Can you work these out from the model? Positions are in its coordinate system, mm. Coordinates: 2 decimals unless noted, no trailing zeros. Write each loop counter-clockwise with the first axis right and the second up, starting at its lowest first coordinate (ties: lowest second). Pieces come first, ordered by that corner, then holes. Notation, with made-up numbers: (-20, 81.5) -> (25, 81.5) arc R26 ccw to (25, 98.5) -> close; hole circle Ø6 at (-26, -16.75). An arc over 180 degrees is marked (long way). Use one line per item in the form item = value.
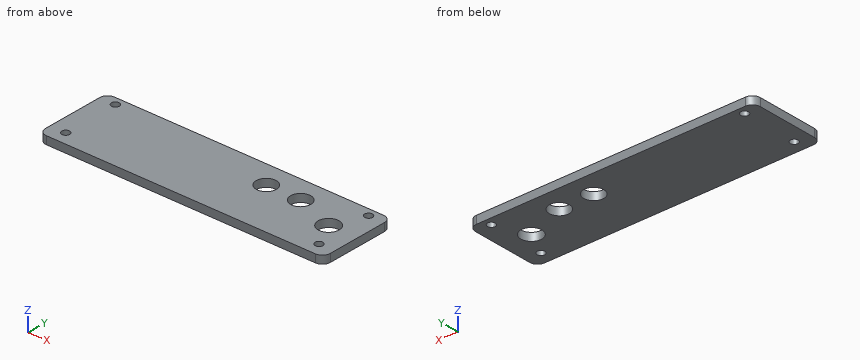
```python
from build123d import *

# Parameters (mm, degrees)
F0_R     = 1.5
F0_R_2   = 3.825
F1_DEPTH = 3


with BuildPart() as f1:
    # F0 (on Top) → F1 (new body)
    with BuildSketch(Plane.XY):
        with BuildLine():
            Line((54.25, -11.75), (54.25, 0))
            Line((54.25, 0), (47.317251, 0))
            ThreePointArc((47.317251, 0), (43.317251, -4), (39.317251, 0))
            Line((39.317251, 0), (-54.25, 0))
            Line((-54.25, 0), (-54.25, -11.75))
            ThreePointArc((-54.25, -11.75), (-53.37132, -13.87132), (-51.25, -14.75))
            Line((-51.25, -14.75), (51.25, -14.75))
            ThreePointArc((51.25, -14.75), (53.37132, -13.87132), (54.25, -11.75))
        make_face()
        with Locations((-48.25, -9.8)):
            Circle(F0_R, mode=Mode.SUBTRACT)
        with Locations((48.25, -9.8)):
            Circle(F0_R, mode=Mode.SUBTRACT)
        with BuildLine():
            ThreePointArc((54.25, 11.75), (53.37132, 13.87132), (51.25, 14.75))
            Line((51.25, 14.75), (-51.25, 14.75))
            ThreePointArc((-51.25, 14.75), (-53.37132, 13.87132), (-54.25, 11.75))
            Line((-54.25, 11.75), (-54.25, 0))
            Line((-54.25, 0), (39.317251, 0))
            ThreePointArc((39.317251, 0), (43.317251, 4), (47.317251, 0))
            Line((47.317251, 0), (54.25, 0))
            Line((54.25, 0), (54.25, 11.75))
        make_face()
        with Locations((-48.25, 11.7)):
            Circle(F0_R, mode=Mode.SUBTRACT)
        with Locations((14.629073, 5.604644)):
            Circle(F0_R_2, mode=Mode.SUBTRACT)
        with Locations((27.738241, 5.604644)):
            Circle(F0_R_2, mode=Mode.SUBTRACT)
        with Locations((48.25, 11.7)):
            Circle(F0_R, mode=Mode.SUBTRACT)
    extrude(amount=F1_DEPTH)


solid = f1.part
```
Q1. Will this pin go through, and if not, where does the flat tip stop? pin 1 (6.5 mm diameter, centred on x = 43.32, y = 0, fed in from -Z).
Return value:
pin_1 = through
Q2. Suppose I cut it at D-D (x = 14). Write out the boundary of the cut face in (y, z).
Return value:
outline = (-14.75, 0) -> (1.83, 0) -> (1.83, 3) -> (-14.75, 3) -> close; (9.38, 0) -> (14.75, 0) -> (14.75, 3) -> (9.38, 3) -> close
Q3. Suppose I cut it at B-B (y = -9.8). Write out the boundary of the cut face in (x, z), then the cut area to 4 significant figures.
Return value:
outline = (-54.25, 0) -> (-49.75, 0) -> (-49.75, 3) -> (-54.25, 3) -> close; (-46.75, 0) -> (46.75, 0) -> (46.75, 3) -> (-46.75, 3) -> close; (49.75, 0) -> (54.25, 0) -> (54.25, 3) -> (49.75, 3) -> close
area = 307.5 mm2
Q4. Suppose I cut it at A-A (y = 0). Write out the boundary of the cut face in (x, z), then the cut area to 4 significant figures.
Return value:
outline = (-54.25, 0) -> (39.32, 0) -> (39.32, 3) -> (-54.25, 3) -> close; (47.32, 0) -> (54.25, 0) -> (54.25, 3) -> (47.32, 3) -> close
area = 301.5 mm2
Q5. Suppose I cut it at C-C (x = 48.25). Write out the boundary of the cut face in (y, z).
Return value:
outline = (-14.75, 0) -> (-11.3, 0) -> (-11.3, 3) -> (-14.75, 3) -> close; (-8.3, 0) -> (10.2, 0) -> (10.2, 3) -> (-8.3, 3) -> close; (13.2, 0) -> (14.75, 0) -> (14.75, 3) -> (13.2, 3) -> close
Q6. If I drill on line 1 (Y direction, x = -48.25, z = 2.2); line 2 (X direction, y = -10, z = 2.9); line 3 (X direction, y = -10.75, z = 0.8), over which ranges is the centre line in solid material (lowest first)? Write a range as from..to.
Return value:
line_1 = -14.75..-11.3, -8.3..10.2, 13.2..14.75
line_2 = -54.25..-49.74, -46.76..46.76, 49.74..54.25
line_3 = -54.25..-49.41, -47.09..47.09, 49.41..54.25
